Read the model definition and answer for the solid it produces. Units are mm, in the model's axes. Face numbers are marked on the shaded views. A direction names the side the tool comes from. Coordinates: 2 decimals unless noted, no trailing zeros.
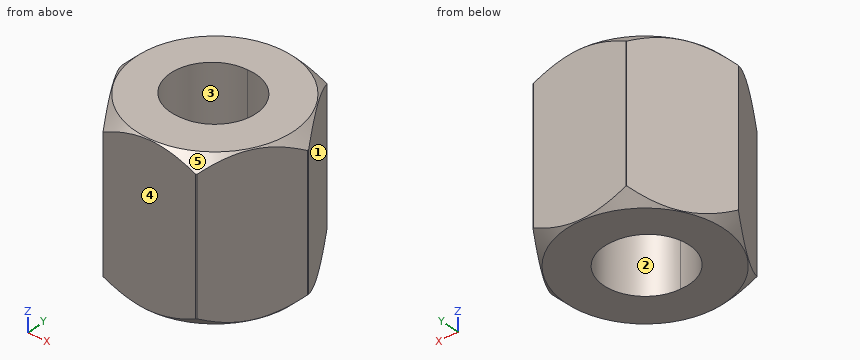
Autodesk Inventor part; units mm, degrees
ref_plane "Work Plane1" through (-1.711, 0.0003, 0) normal (0, 1, 0) x (1, 0, 0)
ref_plane "Work Plane2" through (0.1135, 0.0003, 3.175) normal (0, 0, -1) x (-1, 0, 0)
ref_plane "YZ Plane" through (0, 0, 0) normal (1, 0, 0) x (0, 1, 0)
sketch "Sketch1" plane through (0, 0, 0) normal (0, 0, 1) x (1, 0, 0)
  line L0 (1.9552, -3.1747) -> (-1.711, -3.1747)
  line L1 (-1.711, -3.1747) -> (-3.5441, 0.0003)
  line L2 (-3.5441, 0.0003) -> (-1.711, 3.1753)
  line L3 (-1.711, 3.1753) -> (1.9552, 3.1753)
  line L4 (1.9552, 3.1753) -> (3.7883, 0.0003)
  line L5 (3.7883, 0.0003) -> (1.9552, -3.1747)
  point P0 (0.1221, 0.0003)
  dimension "d0" = 6.35
extrude "Extrusion1" add sketch "Sketch1" along normal blind 6.35
ref_plane "Work Plane1" through (-1.711, 0.0003, 0) normal (0, 1, 0) x (1, 0, 0)
sketch "Sketch3" plane through (-1.711, 0.0003, 0) normal (0, 1, 0) x (1, 0, 0)
  line L0 (-1.3251, 0) -> (4.9741, 0)
  line L1 (5.4821, -0.508) -> (5.4821, -5.842)
  line L2 (-1.8331, -5.842) -> (-1.8331, -0.508)
  line L3 (-1.8331, -0.508) -> (-1.3251, 0)
  line L4 (4.9741, 0) -> (5.4821, -0.508)
  line L5 (-1.8331, 0) -> (-1.8331, -6.35)
  line L6 (3.6662, 0) -> (5.4993, 0)
  line L7 (1.8245, 0) -> (1.8245, -6.35)
  line L8 (0, -6.35) -> (-1.8331, -6.35)
  line L9 (5.4993, -6.35) -> (3.6662, -6.35)
  line L10 (3.6662, -6.35) -> (0, -6.35)
  line L11 (-1.3251, -6.35) -> (-1.8331, -5.842)
  line L12 (4.9741, -6.35) -> (5.4821, -5.842)
  point P0 (-1.8331, 0)
  point P1 (5.4821, 0)
  point P2 (5.4821, -6.35)
  dimension "d5" = 0.508
  dimension "d6" = 0.508
  dimension "d7" = 0.508
  dimension "d8" = 0.508
  dimension "d16" = 0
  dimension "d46" = 0.508
  dimension "d47" = 0.508
  dimension "d48" = 0.508
  dimension "d49" = 0.508
revolve "Revolution1" cut sketch "Sketch3" angle 360 about axis through (0.1135, 0.0003, 0) along (0, 0, 1) keep common part contours L0 L4 L1 L12 L9 L10 L7
sketch "Sketch6" plane through (0.1135, 0.0003, 0) normal (0, 0, -1) x (-1, 0, 0)
  circle A0 centre (0, 0) radius 3.1496
hole "Hole3" at (0.1135, 0.0003, 0) direction (0, 0, 1) diameter 3.302 depth 6.35 tip angle 118
sketch "Sketch7" plane through (0, 0, 6.35) normal (0, 0, 1) x (1, 0, 0)
  point P0 (0, 0)
hole "Hole4" at (0, 0, 6.35) direction (0, 0, -1) diameter 3.302 depth 6.35 tip angle 118
ref_plane "Work Plane2" through (0.1135, 0.0003, 3.175) normal (0, 0, -1) x (-1, 0, 0)
properties part number "0.25 inch Standoff" material "Steel"
Q1. Determine the mould class of the marked faces 3, 4 and 5 for opening direction X: +X half, -X half, draft (parallel to the pull), parting line (faces both ways), or undercut.
Q2. Which of the six approach directions +Z, -Z, +X, -X, +Y, -Y give full straight-line access (tool end or side, diameter ignored) to the marked faces 1 and 2?
Q3. Each of these flat-tipped pins is pushed along its axis until it touches: P1, Ø2, axis at y = 2.5, z = 5, coming from the +X side; P2, Ø1.5, axis at x = 2, z = 2.5, coming from the -Y side; P3, Ø1, axis at y = -1, z = 1, coming from the -X side. Where does it stop, or does it pass through?
Q4. Straight lines are drawn through the part: L1, parallel to Y at x = -0.75, z = 2.75; L2, parallel to X at y = 0.5, z = 5.75; L3, parallel to X at y = 0.25, z = 6. For each, find the intervals that lie inside material, in ascending order.
Computed values:
1. face 3: undercut
1. face 4: draft
1. face 5: parting line
2. face 1: +Z, -Z, +X, +Y
2. face 2: +Z, -Z
3. P1: stops at x = 2.92
3. P2: stops at y = -3.17
3. P3: stops at x = -3.26
4. L1: y = -3.17 to -1.47, 1.47 to 3.18
4. L2: x = -3.26 to -1.57, 1.69 to 3.5
4. L3: x = -3.38 to -1.63, 1.75 to 3.6
